from build123d import *

# Parameters (mm, degrees)
SZKIC2_W                           = 16.5
SZKIC2_H                           = 6.75
ODGI_CIE_BAZOWE1_DEPTH             = 0.75
ODGI_CIE_KRAW_DZI1_STRIP_W         = 7
ODGI_CIE_KRAW_DZI1_STRIP_H         = 0.75
ODGI_CIE_KRAW_DZI1_STRIP_CUT_DEPTH = 6.75
ODGI_CIE_KRAW_DZI1_DEPTH           = 6.75
ODGI_CIE_KRAW_DZI2_STRIP_W         = 7
ODGI_CIE_KRAW_DZI2_STRIP_H         = 0.75
ODGI_CIE_KRAW_DZI2_STRIP_CUT_DEPTH = 6.75
ODGI_CIE_KRAW_DZI2_DEPTH           = 6.75
SZKIC16_W                          = 18.3
SZKIC16_H                          = 1.55
DODANIE_WYCI_GNI_CIE2_DEPTH        = 1.55
DODANIE_WYCI_GNI_CIE3_DEPTH        = 1.55
SZKIC19_R                          = 0.95
WYTNIJ_WYCI_GNI_CIE1_DEPTH         = 0.75


# Sheet-metal steps are written as plain solids
with BuildPart() as part:
    # Szkic2 → Odgięcie bazowe1 (new body)
    with BuildSketch(Plane(origin=(0, 0, 0), x_dir=(0, 0, -1), z_dir=(1, 0, 0))):
        with Locations((-5.0166528, -4.366319951)):
            Rectangle(SZKIC2_W, SZKIC2_H)
    extrude(amount=-ODGI_CIE_BAZOWE1_DEPTH)

    # Odgięcie krawędzi1 strip (across the edge) → Odgięcie krawędzi1 strip cut (cut)
    with BuildSketch(Plane(origin=(-0.75, -7.741319951, 13.2666528), x_dir=(0, 0, -1), z_dir=(0, 1, 0))):
        with Locations((-0.75, -0.375)):
            Rectangle(ODGI_CIE_KRAW_DZI1_STRIP_W, ODGI_CIE_KRAW_DZI1_STRIP_H)
    extrude(amount=ODGI_CIE_KRAW_DZI1_STRIP_CUT_DEPTH, mode=Mode.SUBTRACT)

    # Odgięcie krawędzi1 section (across the edge) → Odgięcie krawędzi1 (add)
    with BuildSketch(Plane(origin=(-0.75, -7.741319951, 13.2666528), x_dir=(0, 0, -1), z_dir=(0, 1, 0))):
        with BuildLine():
            Line((0, 2), (0, 6.75))
            Line((0, 6.75), (0.75, 6.75))
            Line((0.75, 6.75), (0.75, 2))
            ThreePointArc((0.75, 2), (1.335786438, 0.585786438), (2.75, 0))
            Line((2.75, 0), (2.75, -0.75))
            ThreePointArc((2.75, -0.75), (0.805456352, 0.055456352), (0, 2))
        make_face()
    extrude(amount=ODGI_CIE_KRAW_DZI1_DEPTH)

    # Odgięcie krawędzi2 strip (across the edge) → Odgięcie krawędzi2 strip cut (cut)
    with BuildSketch(Plane(origin=(-0.75, -0.991319951, -3.2333472), x_dir=(0, 0, 1), z_dir=(0, -1, 0))):
        with Locations((-0.75, -0.375)):
            Rectangle(ODGI_CIE_KRAW_DZI2_STRIP_W, ODGI_CIE_KRAW_DZI2_STRIP_H)
    extrude(amount=ODGI_CIE_KRAW_DZI2_STRIP_CUT_DEPTH, mode=Mode.SUBTRACT)

    # Odgięcie krawędzi2 section (across the edge) → Odgięcie krawędzi2 (add)
    with BuildSketch(Plane(origin=(-0.75, -0.991319951, -3.2333472), x_dir=(0, 0, 1), z_dir=(0, -1, 0))):
        with BuildLine():
            Line((0, 2), (0, 15))
            Line((0, 15), (0.75, 15))
            Line((0.75, 15), (0.75, 2))
            ThreePointArc((0.75, 2), (1.335786438, 0.585786438), (2.75, 0))
            Line((2.75, 0), (2.75, -0.75))
            ThreePointArc((2.75, -0.75), (0.805456352, 0.055456352), (0, 2))
        make_face()
    extrude(amount=ODGI_CIE_KRAW_DZI2_DEPTH)

    # Szkic16 → Dodanie-wyciągnięcie2 (add)
    with BuildSketch(Plane(origin=(0, 0, -3.2333472), x_dir=(-1, 0, 0), z_dir=(0, 0, -1))):
        with Locations((9.15, -4.636679938)):
            Rectangle(SZKIC16_W, SZKIC16_H)
    extrude(amount=DODANIE_WYCI_GNI_CIE2_DEPTH)

    # Szkic18 → Dodanie-wyciągnięcie3 (add)
    with BuildSketch(Plane(origin=(0, -3.861679938, 0), x_dir=(1, 0, 0), z_dir=(0, 1, 0))):
        Polygon((-45.013147785, 15.032481597), (-54.013147785, 15.032481597), (-54.013147785, -15.585696439), (-52.463147785, -15.585696439), (-52.463147785, 9.864303561), (-45.013147785, 9.864303561), (-43.64142473, 8.982481597), (-20.713147785, 8.982481597), (-18.3, 3.2333472), (-18.3, 4.7833472), (-20.713147785, 10.532481597), (-38.013147785, 10.532481597), align=None)
    extrude(amount=-DODANIE_WYCI_GNI_CIE3_DEPTH)

    # Szkic19 → Wytnij-wyciągnięcie1 (cut)
    with BuildSketch(Plane(origin=(0, 0, 0), x_dir=(0, 0, -1), z_dir=(1, 0, 0))):
        with Locations((-0.5666528, -4.366319951)):
            Circle(SZKIC19_R)
        with Locations((-9.464367913, -4.366319951)):
            Circle(SZKIC19_R)
    extrude(amount=-WYTNIJ_WYCI_GNI_CIE1_DEPTH, mode=Mode.SUBTRACT)


solid = part.part
Geometry check sheet. Reference: the model listing, model coordinates, mm. A direction names the side the tool comes from. Round coordinates to 2 decimals unless told otherwise and drop trailing zeros. Loops run counter-clockwise (first coordinate to the right, second up) from the corner with the lowest first, then second, coordinate; pieces in that order, holes last. Notation, with made-up numbers: (36, 14) - (68, 14) arc R6 cw to (68, 23) - close; hole circle Ø8 at (82, 42). An arc over 180 degrees is marked (long way). One line per question, with ' | ' between items. Start each with the question number.
1. Cross-section at C-C on y = -2.75. Record the cut outline in (x, z), then the cut area to 3 significant figures.
2. Draft check along X on faces 5 (the face through (-5, -4, 12.517)), 6 (the face through (0, -4, 5)), 7 (the face through (-1.351, -4.414, 11.946)), 8 (the face through (-53, -5, 15.586)). Enter one of: released by +X, released by -X, zero draft, split by the parting line, or undercut.
3. Cross-section at A-A on x = -4. Record the cut outline in (y, z).
4. Scan lines: line 1 (Z direction, x = -3, y = -6.25); line 2 (X direction, y = -5, z = 7.5); line 3 (Z direction, x = -35, y = -5.25). Record each from-to range of solid material in increasing order. Write a range as [from, to].
5. Depth check by flat-ended pin: pin 1 (1.2 mm diameter, centred on x = -8.5, y = -7, fed in from -Z); pin 2 (1.7 mm diameter, centred on x = -28.5, y = -4.5, fed in from -Z); pin 3 (1.4 mm diameter, centred on x = -5.5, y = -5, fed in from +Z). Enter the tip coordinate at first touch or a pass-through.
6. Cross-section at B-B on z = 3.5. Record the cut outline in (x, y), then the cut area to 4 significant figures.
7. Tool access check on faces 1 (the face through (-52.463, -5, 3)), 2 (the face through (-9, -7, -3.233)), 3 (the face through (-9, -5, -4.783)), 4 (the face through (-5, -4, 13.267)). Record the directions out of +Z, -Z, +X, -X, +Y, -Y that give a thin tool (end or side, any length) a straight path to the whole face; none if there is none.
8. Cross-section at D-D on x = -12. Record the cut outline in (y, z), then the cut area to 4 significant figures.
Taken from the geometry:
1) outline: (-15.75, -3.23) - (-2.75, -3.23) arc R2.75 ccw to (0, -0.48) - (0, 10.52) arc R2.75 ccw to (-2.75, 13.27) - (-7.5, 13.27) - (-7.5, 12.52) - (-2.75, 12.52) arc R2 cw to (-0.75, 10.52) - (-0.75, -0.48) arc R2 cw to (-2.75, -2.48) - (-15.75, -2.48) - close | area: 27.2 mm²
2) face 5: undercut | face 6: released by +X | face 7: undercut | face 8: zero draft
3) outline: (-7.74, -3.23) - (-5.41, -3.23) - (-5.41, -4.78) - (-3.86, -4.78) - (-3.86, -3.23) - (-0.99, -3.23) - (-0.99, -2.48) - (-7.74, -2.48) - close; (-7.74, 12.52) - (-0.99, 12.52) - (-0.99, 13.27) - (-7.74, 13.27) - close
4) line 1: [-3.23, -2.48], [12.52, 13.27] | line 2: [-54.01, -52.46], [-0.75, 0] | line 3: [-10.53, -8.98]
5) pin 1: z = -3.23 | pin 2: z = -10.53 | pin 3: z = 13.27
6) outline: (-54.01, -5.41) - (-52.46, -5.41) - (-52.46, -3.86) - (-54.01, -3.86) - close; (-0.75, -7.74) - (0, -7.74) - (0, -0.99) - (-0.75, -0.99) - close | area: 7.465 mm²
7) face 1: +Z, +Y, -Y | face 2: -Z, +X, -X, -Y | face 3: -Z, +X, +Y, -Y | face 4: +Z, +X, +Y, -Y
8) outline: (-7.74, -3.23) - (-5.41, -3.23) - (-5.41, -4.78) - (-3.86, -4.78) - (-3.86, -3.23) - (-0.99, -3.23) - (-0.99, -2.48) - (-7.74, -2.48) - close | area: 7.465 mm²
